The listing builds one solid part. Answer for the finished solid, in the listing's coordinates (mm). Face numbers are marked on the shaded views. Coordinates: 2 decimals unless noted, no trailing zeros. Write each loop counter-clockwise with the first axis right and the second up, starting at its lowest first coordinate (ties: lowest second). Pieces come first, ordered by that corner, then holes.
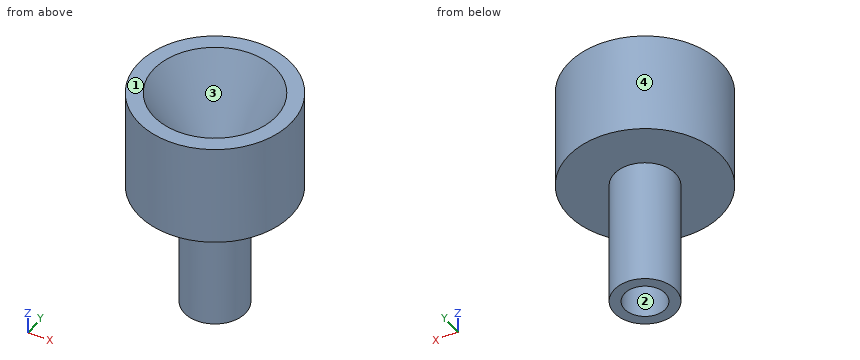
from build123d import *

# Parameters (mm, degrees)
F0_R     = 15
F0_R_2   = 4
F1_DEPTH = 20
F2_SIZE2 = 8
F2_SIZE  = 15
F3_R     = 6
F3_R_2   = 4
F4_DEPTH = 25


with BuildPart() as f1:
    # F0 (on Top) → F1 (new body)
    with BuildSketch(Plane.XY):
        Circle(F0_R)
        Circle(F0_R_2, mode=Mode.SUBTRACT)
    extrude(amount=F1_DEPTH)

    # F2
    f2_edges = [f1.edges().sort_by_distance(p)[0] for p in [
        (-4, 0, 20),
    ]]
    chamfer(f2_edges, length=F2_SIZE, length2=F2_SIZE2)

    # F3 (on face) → F4 (join)
    with BuildSketch(Plane(origin=(0, 0, 0), x_dir=(1, 0, 0), z_dir=(0, 0, -1))):
        Circle(F3_R)
        Circle(F3_R_2, mode=Mode.SUBTRACT)
    extrude(amount=F4_DEPTH)


solid = f1.part
Q1. The part is cut by section C-C, the plane z = 9. Write down the section's boundary in (x, y), then the cut area to 3 significant figures.
Answers below:
outline: circle Ø30 at (0, 0); hole circle Ø12.27 at (0, 0)
area: 589 mm2
Q2. Find the intervals of material crossed by probe 1 along X at (y, z) = (0, -13.5); probe 2 along Z at (x, y) = (-11.25, 5.75), in increasing order.
Answers below:
probe 1: x = -6 to -4, 4 to 6
probe 2: z = 0 to 20
Q3. Determine the mould class of the marked faces 1, 2, 3 and 4 for opening direction Y: released by +Y, released by -Y, zero draft, split by the parting line, or undercut.
Answers below:
face 1: zero draft
face 2: undercut
face 3: undercut
face 4: split by the parting line
Q4. Given pin 1 (5 mm diameter, centred on x = -6, z = -3, fed in from +Y); pin 2 (12 mm diameter, centred on x = -3, y = 6.5, fed in from +Z); pin 3 (6.5 mm diameter, centred on x = 0, y = 0, fed in from -Z); pin 4 (4 mm diameter, centred on y = -7.5, z = -6, fed in from +X), each flat-ended and moving along its own axis, determine where each tip first touches the part or whether it passes through.
Answers below:
pin 1: stops at y = 4.87
pin 2: stops at z = 20
pin 3: passes through
pin 4: stops at x = 2.4
Q5. The part is cut by section A-A, the plane x = 0. Write down the section's boundary in (y, z), then the cut area to 3 significant figures.
Answers below:
outline: (-15, 0) - (-6, 0) - (-6, -25) - (-4, -25) - (-4, 5) - (-12, 20) - (-15, 20) - close; (4, -25) - (6, -25) - (6, 0) - (15, 0) - (15, 20) - (12, 20) - (4, 5) - close
area: 420 mm2
Q6. The part is cut by section D-D, the plane x = -12.75. Write down the section's boundary in (y, z).
Answers below:
outline: (-7.9, 0) - (7.9, 0) - (7.9, 20) - (-7.9, 20) - close
